Here's how the part is built. I have some questions about the finished solid (model axes, mm). A direction names the side the tool comes from. Round coordinates to 2 decimals unless told otherwise and drop trailing zeros. Write each loop counter-clockwise with the first axis right and the second up, starting at its lowest first coordinate (ties: lowest second). Pieces come first, ordered by that corner, then holes. Notation, with made-up numbers: (-13, -27.75) -> (0, -27.75) arc R19 cw to (0, 1.25) -> close; hole circle Ø9 at (-28.5, 56.5). An arc over 180 degrees is marked (long way). Put each result on its own line as item: value. Start each with the question number.
1. Which directions (+Z, -Z, +X, -X, +Y, -Y) give clear straight access to the entire face, cutting with the end or side of a thin tool? Please do faces 1 (the face through (22.9, 36.5, 2.3)), 2 (the face through (51.777, -61.33, 2.342)).
2. Suppose I cut it at B-B (y = 19.05). Please give me the cut outline in (x, z), then the cut area to 3 significant figures.
3. Suppose I cut it at D-D (y = -37.5). Please give me the cut outline in (x, z).
4. Suppose I cut it at C-C (x = -48). Please give me the cut outline in (y, z), then the cut area to 3 significant figures.
5. We'd pull the mould along Y, two halves only. Please class faces 3 (the face through (-2, 49.2, 2.3)), 4 (the face through (-31.073, -11.097, 2.342)), 5 (the face through (-0.299, 45.634, 2.342)), 6 (the face through (8, -4, 4.75)): +Y half, -Y half, draft (parallel to the pull), parting line (faces both ways), or undercut.
6. I need wall thicknesses on probe 1 along Y at (x, z) = (-4.5, 0.4); probe 2 along X at (y, z) = (2.5, 0.65); probe 3 along X at (y, z) = (3, 0.65). Which ranges of each line are inside material? Lowest first, please. Write a range as from..to.
7. For pin 1 (6 mm diameter, centred on x = -2.07, y = 42.85, fed in from -Z); pin 2 (15 mm diameter, centred on x = 47.15, y = 0, fed in from -Z), each with a flat end and sliding along its axis, tell me the tip position at first contact or that it passes through.
8. Suppose I cut it at A-A (z = 3.4). Count the separate pieces of the cut face and the enclosed holes in it, then the cut area to 3 significant figures.
```python
from build123d import *

# Parameters (mm, degrees)
F0_R     = 4.7625
F0_R_2   = 3.302
F1_DEPTH = 4.7498


with BuildPart() as f1:
    # F0 (on Top) → F1 (new body)
    with BuildSketch(Plane.XY):
        with BuildLine():
            Line((44.185468, 24.926487), (0.958828, 48.42856))
            ThreePointArc((0.958828, 48.42856), (-2.042016, 49.199718), (-5.050549, 48.459123))
            Line((-5.050549, 48.459123), (-46.477872, 26.478292))
            ThreePointArc((-46.477872, 26.478292), (-48.186948, 25.277873), (-49.547481, 23.69329))
            Line((-49.547481, 23.69329), (-61.470053, 5.69123))
            ThreePointArc((-61.470053, 5.69123), (-63.1567, -3.061793), (-55.904223, -8.244627))
            Line((-55.904223, -8.244627), (-30.697283, -9.509502))
            Line((-30.697283, -9.509502), (-31.459969, -12.728965))
            Line((-31.459969, -12.728965), (-19.071049, -15.525871))
            Line((-19.071049, -15.525871), (-18.340647, -12.442686))
            ThreePointArc((-18.340647, -12.442686), (-9.722602, -18.326584), (-3.477553, -26.686626))
            Line((-3.477553, -26.686626), (39.618722, -85.851888))
            ThreePointArc((39.618722, -85.851888), (50.31508, -90.098295), (54.861639, -79.526027))
            Line((54.861639, -79.526027), (48.604056, -42.618147))
            ThreePointArc((48.604056, -42.618147), (48.489523, -41.145608), (48.641425, -39.676454))
            Line((48.641425, -39.676454), (55.284238, -1.41197))
            ThreePointArc((55.284238, -1.41197), (55.336524, 1.067899), (54.649768, 3.451354))
            Line((54.649768, 3.451354), (45.771288, 22.741944))
            ThreePointArc((45.771288, 22.741944), (45.068278, 23.899477), (44.185468, 24.926487))
        make_face()
        with Locations((47.150889, -82.4738)):
            Circle(F0_R, mode=Mode.SUBTRACT)
        with Locations((-55.490511, 0)):
            Circle(F0_R, mode=Mode.SUBTRACT)
        with Locations((-42.536511, 19.05)):
            Circle(F0_R_2, mode=Mode.SUBTRACT)
        with Locations((-2.074311, -0.762)):
            Circle(F0_R, mode=Mode.SUBTRACT)
        with Locations((47.150889, 0)):
            Circle(F0_R, mode=Mode.SUBTRACT)
        with Locations((-2.074311, 42.8498)):
            Circle(F0_R_2, mode=Mode.SUBTRACT)
        with Locations((38.387889, 19.05)):
            Circle(F0_R_2, mode=Mode.SUBTRACT)
    extrude(amount=F1_DEPTH)


solid = f1.part
```
Verdict:
1. face 1: +Z, -Z, +X, +Y
1. face 2: +Z, -Z, +X
2. outline: (-52.62, 0) -> (-45.84, 0) -> (-45.84, 4.75) -> (-52.62, 4.75) -> close; (-39.23, 0) -> (35.09, 0) -> (35.09, 4.75) -> (-39.23, 4.75) -> close; (41.69, 0) -> (47.47, 0) -> (47.47, 4.75) -> (41.69, 4.75) -> close
2. area: 413 mm^2
3. outline: (4.4, 0) -> (49.02, 0) -> (49.02, 4.75) -> (4.4, 4.75) -> close
4. outline: (-8.64, 0) -> (25.44, 0) -> (25.44, 4.75) -> (-8.64, 4.75) -> close
4. area: 162 mm^2
5. face 3: +Y half
5. face 4: undercut
5. face 5: undercut
5. face 6: draft
6. probe 1: y = -24.86..-4.86, 3.34..40.61, 45.09..48.72
6. probe 2: x = -63.36..-59.54, -51.44..-5.54, 1.4..43.1, 51.2..55.02
6. probe 3: x = -63.18..-59.19, -51.79..-4.99, 0.85..43.45, 50.85..54.84
7. pin 1: passes through
7. pin 2: stops at z = 0
8. separate pieces: 1
8. enclosed holes: 7
8. area: 7,720 mm^2
